from build123d import *

# Parameters (mm, degrees)
F0_R             = 22.225
F0_R_2           = 2.15265
F1_DEPTH         = 12.7
F3_DEPTH         = 12.7
F4_COUNT         = 6
F4_ANGLE         = 300
F6_R             = 11.90625
F7_DEPTH         = 11.47445
F10_R            = 3.96875
F11_DEPTH        = 9.525
F12_R            = 3.96875
F13_DEPTH        = 9.525
F15_DEPTH        = 12.7
F15_COPIES_COUNT = 4


# Not quite as in the source:
# - a pattern or mirror of a feature is missing from the dataset's text; its kind, count and spacing are read off the source's solid


with BuildPart() as f1:
    # F0 (on Top) → F1 (new body)
    with BuildSketch(Plane.XY):
        Circle(F0_R)
        with Locations((-11.7865861589, -11.7865861589)):
            Circle(F0_R_2, mode=Mode.SUBTRACT)
        with Locations((11.7865861589, -11.7865861589)):
            Circle(F0_R_2, mode=Mode.SUBTRACT)
        with Locations((-11.7865861589, 11.7865861589)):
            Circle(F0_R_2, mode=Mode.SUBTRACT)
        with BuildLine():
            ThreePointArc((0, 11.1125), (7.8577241059, 7.8577241059), (11.1125, 0))
            ThreePointArc((11.1125, 0), (-7.8577241059, -7.8577241059), (0, 11.1125))
        make_face(mode=Mode.SUBTRACT)
        with Locations((11.7865861589, 11.7865861589)):
            Circle(F0_R_2, mode=Mode.SUBTRACT)
    extrude(amount=F1_DEPTH)

    # F2 (on face) → F3 (cut, through all)
    with BuildSketch(Plane.XY.offset(12.7)):
        with BuildLine():
            ThreePointArc((-2.8761266387, 10.7338507446), (0, 11.1125), (2.8761266387, 10.7338507446))
            Line((2.8761266387, 10.7338507446), (3.0815642558, 11.5005543693))
            ThreePointArc((3.0815642558, 11.5005543693), (0, 11.90625), (-3.0815642558, 11.5005543693))
            Line((-3.0815642558, 11.5005543693), (-2.8761266387, 10.7338507446))
        make_face()
    f3 = extrude(amount=-F3_DEPTH, mode=Mode.SUBTRACT)

    # F4: F3 ×6 about axis
    f4_axis = Axis((0, 0, 0), (0, 0, -1))
    for i in range(1, F4_COUNT):
        add(f3.rotate(f4_axis, i * F4_ANGLE / (F4_COUNT - 1)), mode=Mode.SUBTRACT)

    # F6 (on face) → F7 (cut, through all)
    with BuildSketch(Plane(origin=(0, 0, 0), x_dir=(1, 0, 0), z_dir=(0, 0, -1))):
        Circle(F6_R)
    extrude(amount=-F7_DEPTH, mode=Mode.SUBTRACT)

    # F10 (on face) → F11 (cut, through all)
    with BuildSketch(Plane(origin=(0, 0, 0), x_dir=(1, 0, 0), z_dir=(0, 0, -1))):
        with Locations((11.7865861589, -11.7865861589)):
            Circle(F10_R)
        with Locations((-11.7865861589, 11.7865861589)):
            Circle(F10_R)
    extrude(amount=-F11_DEPTH, mode=Mode.SUBTRACT)

    # F12 (on face) → F13 (cut, through all)
    with BuildSketch(Plane.XY.offset(12.7)):
        with Locations((-11.7865861589, 11.7865861589)):
            Circle(F12_R)
        with Locations((11.7865861589, -11.7865861589)):
            Circle(F12_R)
    extrude(amount=-F13_DEPTH, mode=Mode.SUBTRACT)

    # F14 (on face) → F15 (cut, through all)
    with BuildSketch(Plane(origin=(0, 0, 0), x_dir=(1, 0, 0), z_dir=(0, 0, -1))):
        with BuildLine():
            ThreePointArc((-11.229543123, 17.3148424047), (-8.3361072587, 16.1415958514), (-6.5322351826, 13.5931602316))
            ThreePointArc((-6.5322351826, 13.5931602316), (0, 15.08125), (6.5322351826, 13.5931602316))
            ThreePointArc((6.5322351826, 13.5931602316), (8.3361072587, 16.1415958514), (11.229543123, 17.3148424047))
            ThreePointArc((11.229543123, 17.3148424047), (0, 20.6375), (-11.229543123, 17.3148424047))
        make_face()
    f15 = extrude(amount=-F15_DEPTH, mode=Mode.SUBTRACT)

    # F15_copies: F15 ×4 about axis
    f15_copies_axis = Axis((0, 0, 0), (0, 0, 1))
    for i in range(1, F15_COPIES_COUNT):
        add(f15.rotate(f15_copies_axis, i * 360 / F15_COPIES_COUNT), mode=Mode.SUBTRACT)


solid = f1.part
Design review of the part built by this model. Coordinates are the model's own, in mm. A direction names the side the tool comes from. Give positions to 0.01 mm unless a question says otherwise; leave off trailing zeros. Write each loop counter-clockwise with the first axis right and the second up, starting at its lowest first coordinate (ties: lowest second). Pieces come first, ordered by that corner, then holes. Notation, with made-up numbers: M 69.25,23.5 L 77.25,23.5 A27 ccw 77.25,41.5 Z; hole C -30.75,-33 d1. An arc over 180 degrees is marked long. Return JSON: item names as keys, results as strings. Group by question number.
Item 1: Tool access review of faces 1 (the cylindrical face through (-5.6, 9.6, 12.1)), 2 (the flat face through (-10, -10, 9.525)), 3 (the cylindrical face through (15.45, -13.31, 8)): name each direction out of +Z, -Z, +X, -X, +Y, -Y from which nothing blocks a thin tool from reaching the whole face with its end or side.
Item 2: Wall thickness on line 1 along X through (y, z) = (-5, 5); line 2 along X through (y, z) = (13, 10.75); line 3 along X through (y, z) = (9, 6.75): over which ranges is each line inside the solid? List them lowest first.
Item 3: Take a section at B-B (z = 5). Count the separate pieces of the cut face and the enclosed holes in it, plus the area to 3 significant figures.
Item 4: The part is to be moulded in two halves that separate along X. For faces 4 (the cylindrical face through (-16.17, 8.37, 6.26)), 5 (the cylindrical face through (0.09, 15.08, 6.26)), say which applies: pulls with the +X half, pulls with the -X half, needs draft (parallel to the pull), parting line crosses it, or undercut.
Item 5: Take a section at C-C (x = -19.5). Give the boundary of the cut face in (y, z), plus the area to 3 significant figures.
Item 6: Take a section at A-A (x = 0). Give the boundary of the cut face in (y, z) (1 decimal).
Item 7: Clearance check with flat-ended pins moving along their axes: pin 1 Ø3 at (y, z) = (16, 4) entering from -X; pin 2 Ø2.5 at (x, y) = (13.5, 10.5) entering from -Z (3 decimals); pin 3 Ø1.8 at (x, y) = (5.5, -9) entering from -Z. State where each tip first meets the part, or that it passes through.
Item 8: Take a section at D-D (y = -1). Give the boundary of the cut face in (x, z).
Return value:
{
 "1": {"face 1": "+Z, -Z", "face 2": "-Z", "face 3": "+Z"},
 "2": {"line 1": "x = -21.66 to -20.02, -14.23 to -10.81, 10.81 to 14.23, 20.02 to 21.66", "line 2": "x = -18.03 to -15.57, -8.01 to 10.01, 13.56 to 18.03", "line 3": "x = -20.32 to -18.57, -16.59 to -14.61, -8.96 to -7.79, 7.79 to 8.96, 14.61 to 16.59, 18.57 to 20.32"},
 "3": {"separate pieces": "1", "enclosed holes": "9", "area": "523 mm2"},
 "4": {"face 4": "undercut", "face 5": "undercut"},
 "5": {"outline": "M -10.66,0 L -6.76,0 L -6.76,12.7 L -10.66,12.7 Z; M 6.76,0 L 10.66,0 L 10.66,12.7 L 6.76,12.7 Z", "area": "99.2 mm2"},
 "6": {"outline": "M -22.2,0 L -20.6,0 L -20.6,12.7 L -22.2,12.7 Z; M -15.1,0 L -11.9,0 L -11.9,12.7 L -15.1,12.7 Z; M 11.9,0 L 15.1,0 L 15.1,12.7 L 11.9,12.7 Z; M 20.6,0 L 22.2,0 L 22.2,12.7 L 20.6,12.7 Z"},
 "7": {"pin 1": "stops at x = -16.84", "pin 2": "stops at z = 9.525", "pin 3": "stops at z = 11.47"},
 "8": {"outline": "M -22.2,0 L -20.61,0 L -20.61,12.7 L -22.2,12.7 Z; M -15.05,0 L -11.86,0 L -11.86,11.47 L -11.07,11.47 L -11.07,12.7 L -15.05,12.7 Z; M 11.07,11.47 L 11.86,11.47 L 11.86,0 L 15.05,0 L 15.05,12.7 L 11.07,12.7 Z; M 20.61,0 L 22.2,0 L 22.2,12.7 L 20.61,12.7 Z"}
}
